Geometry: final body of the model. Coordinates: model frame, mm. Give positions to 0.01 mm unless a question says otherwise; leave off trailing zeros. Order: outer loops, then holes, each group sorted by start corner. A loop starts at its lowest first (then second) coordinate and runs counter-clockwise, first axis right, second up. Notation, with made-up numbers: (6, -38) -> (28, -38) arc R24 cw to (28, -15) -> close; hole circle Ø3 at (79, -26.75). An arc over 180 degrees is marked (long way). Write item = value, one per line.
```python
from build123d import *

# Parameters (mm, degrees)
SKETCH1_W                        = 250
SKETCH1_H                        = 250
BOSS_EXTRUDE1_DEPTH              = 50
SKETCH2_W                        = 40
SKETCH2_H                        = 100
SKETCH2_H_2                      = 50
CUT_EXTRUDE1_DEPTH               = 45
FILLET1_R                        = 5
FILLET2_R                        = 5
SKETCH5_R                        = 6.25
CUT_EXTRUDE2_DEPTH               = 22
FILLET5_R                        = 1.5
LPATTERN4_COUNT                  = 10
LPATTERN4_PITCH                  = 16.5
LPATTERN4_COUNT_DIR2             = 10
LPATTERN4_PITCH_DIR2             = 16.5
FILLET5_OF_LPATTERN4_R           = 1.5
CUT_EXTRUDE4_DEPTH               = 45
SKETCH8_W                        = 100
SKETCH8_H                        = 20
CUT_EXTRUDE5_DEPTH               = 30
FILLET6_R                        = 2.5
FILLET7_R                        = 2
SKETCH10_R                       = 13.5
CUT_EXTRUDE6_DEPTH               = 358.071421427
SKETCH4_W                        = 25
SKETCH4_H                        = 17.5
CUT_EXTRUDE7_DEPTH               = 10
VERRUNDUNG1_R                    = 2.5
SKIZZE2_W                        = 25
SKIZZE2_H                        = 5
AUFSATZ_LINEAR_AUSTRAGEN1_DEPTH  = 12.5
AUFSATZ_LINEAR_AUSTRAGEN2_DEPTH  = 10
SKIZZE11_W                       = 164
SKIZZE11_H                       = 164
SCHNITT_LINEAR_AUSTRAGEN6_DEPTH  = 10
SKIZZE12_W                       = 174
SKIZZE12_H                       = 174
SCHNITT_LINEAR_AUSTRAGEN7_DEPTH  = 2.5
SKIZZE13_R                       = 1.5
SCHNITT_LINEAR_AUSTRAGEN8_DEPTH  = 2.5
SKIZZE14_W                       = 10
SKIZZE14_H                       = 10
AUFSATZ_LINEAR_AUSTRAGEN3_DEPTH  = 45
SKIZZE16_W                       = 45
SKIZZE16_H                       = 250
SCHNITT_LINEAR_AUSTRAGEN9_DEPTH  = 358.071421427
SKIZZE17_R                       = 2.5
SCHNITT_LINEAR_AUSTRAGEN10_DEPTH = 5
SKIZZE18_W                       = 174.6
SKIZZE18_H                       = 174.6
SCHNITT_LINEAR_AUSTRAGEN11_DEPTH = 2.5
SKIZZE19_W                       = 165
SKIZZE19_H                       = 165
SCHNITT_LINEAR_AUSTRAGEN12_DEPTH = 2.5


with BuildPart() as part:
    # Sketch1 → Boss-Extrude1 (new body)
    with BuildSketch(Plane.XY):
        with Locations((-125, 125)):
            Rectangle(SKETCH1_W, SKETCH1_H)
    extrude(amount=BOSS_EXTRUDE1_DEPTH)

    # Sketch2 → Cut-Extrude1 (cut)
    with BuildSketch(Plane.XY.offset(50)):
        with Locations((-35, 170)):
            Rectangle(SKETCH2_W, SKETCH2_H)
        with Locations((-35, 70)):
            Rectangle(SKETCH2_W, SKETCH2_H_2)
    extrude(amount=-CUT_EXTRUDE1_DEPTH, mode=Mode.SUBTRACT)

    # Fillet1
    fillet1_edges = [part.edges().sort_by_distance(p)[0] for p in [
        (-55, 170, 50),
        (-35, 120, 50),
        (-15, 170, 50),
        (-35, 220, 50),
    ]]
    fillet(fillet1_edges, radius=FILLET1_R)

    # Fillet2
    fillet2_edges = [part.edges().sort_by_distance(p)[0] for p in [
        (-55, 70, 50),
        (-35, 45, 50),
        (-15, 70, 50),
        (-35, 95, 50),
    ]]
    fillet(fillet2_edges, radius=FILLET2_R)

    # Sketch5 → Cut-Extrude2 (cut)
    with BuildSketch(Plane.XY.offset(50)):
        with Locations((-225, 190)):
            Circle(SKETCH5_R)
    cut_extrude2 = extrude(amount=-CUT_EXTRUDE2_DEPTH, mode=Mode.SUBTRACT)

    # Fillet5
    fillet5_edges = [part.edges().sort_by_distance(p)[0] for p in [
        (-231.25, 190, 50),
    ]]
    fillet(fillet5_edges, radius=FILLET5_R)

    # LPattern4: Cut-Extrude2 10 × 10
    with Locations(*[(i * LPATTERN4_PITCH, -j * LPATTERN4_PITCH_DIR2, 0) for i in range(LPATTERN4_COUNT) for j in range(LPATTERN4_COUNT_DIR2) if (i, j) != (0, 0)]):
        add(cut_extrude2, mode=Mode.SUBTRACT)

    # Fillet5 of LPattern4
    fillet5_of_lpattern4_edges = [part.edges().sort_by_distance(p)[0] for p in [
        (-231.25, 173.5, 50),
        (-231.25, 157, 50),
        (-231.25, 140.5, 50),
        (-231.25, 124, 50),
        (-231.25, 107.5, 50),
        (-231.25, 91, 50),
        (-231.25, 74.5, 50),
        (-231.25, 58, 50),
        (-231.25, 41.5, 50),
        (-214.75, 190, 50),
        (-214.75, 173.5, 50),
        (-214.75, 157, 50),
        (-214.75, 140.5, 50),
        (-214.75, 124, 50),
        (-214.75, 107.5, 50),
        (-214.75, 91, 50),
        (-214.75, 74.5, 50),
        (-214.75, 58, 50),
        (-214.75, 41.5, 50),
        (-198.25, 190, 50),
        (-198.25, 173.5, 50),
        (-198.25, 157, 50),
        (-198.25, 140.5, 50),
        (-198.25, 124, 50),
        (-198.25, 107.5, 50),
        (-198.25, 91, 50),
        (-198.25, 74.5, 50),
        (-198.25, 58, 50),
        (-198.25, 41.5, 50),
        (-181.75, 190, 50),
        (-181.75, 173.5, 50),
        (-181.75, 157, 50),
        (-181.75, 140.5, 50),
        (-181.75, 124, 50),
        (-181.75, 107.5, 50),
        (-181.75, 91, 50),
        (-181.75, 74.5, 50),
        (-181.75, 58, 50),
        (-181.75, 41.5, 50),
        (-165.25, 190, 50),
        (-165.25, 173.5, 50),
        (-165.25, 157, 50),
        (-165.25, 140.5, 50),
        (-165.25, 124, 50),
        (-165.25, 107.5, 50),
        (-165.25, 91, 50),
        (-165.25, 74.5, 50),
        (-165.25, 58, 50),
        (-165.25, 41.5, 50),
        (-148.75, 190, 50),
        (-148.75, 173.5, 50),
        (-148.75, 157, 50),
        (-148.75, 140.5, 50),
        (-148.75, 124, 50),
        (-148.75, 107.5, 50),
        (-148.75, 91, 50),
        (-148.75, 74.5, 50),
        (-148.75, 58, 50),
        (-148.75, 41.5, 50),
        (-132.25, 190, 50),
        (-132.25, 173.5, 50),
        (-132.25, 157, 50),
        (-132.25, 140.5, 50),
        (-132.25, 124, 50),
        (-132.25, 107.5, 50),
        (-132.25, 91, 50),
        (-132.25, 74.5, 50),
        (-132.25, 58, 50),
        (-132.25, 41.5, 50),
        (-115.75, 190, 50),
        (-115.75, 173.5, 50),
        (-115.75, 157, 50),
        (-115.75, 140.5, 50),
        (-115.75, 124, 50),
        (-115.75, 107.5, 50),
        (-115.75, 91, 50),
        (-115.75, 74.5, 50),
        (-115.75, 58, 50),
        (-115.75, 41.5, 50),
        (-99.25, 190, 50),
        (-99.25, 173.5, 50),
        (-99.25, 157, 50),
        (-99.25, 140.5, 50),
        (-99.25, 124, 50),
        (-99.25, 107.5, 50),
        (-99.25, 91, 50),
        (-99.25, 74.5, 50),
        (-99.25, 58, 50),
        (-99.25, 41.5, 50),
        (-82.75, 190, 50),
        (-82.75, 173.5, 50),
        (-82.75, 157, 50),
        (-82.75, 140.5, 50),
        (-82.75, 124, 50),
        (-82.75, 107.5, 50),
        (-82.75, 91, 50),
        (-82.75, 74.5, 50),
        (-82.75, 58, 50),
        (-82.75, 41.5, 50),
    ]]
    fillet(fillet5_of_lpattern4_edges, radius=FILLET5_OF_LPATTERN4_R)

    # Sketch7 → Cut-Extrude4 (cut)
    with BuildSketch(Plane(origin=(0, 0, 0), x_dir=(-1, 0, 0), z_dir=(0, 0, -1))):
        Polygon((5, 245), (245, 245), (245, 5), (5, 5), (5, 40), (60, 40), (60, 100), (5, 100), (5, 115), (60, 115), (60, 225), (5, 225), align=None)
    extrude(amount=-CUT_EXTRUDE4_DEPTH, mode=Mode.SUBTRACT)

    # Sketch8 → Cut-Extrude5 (cut)
    with BuildSketch(Plane.XY.offset(50)):
        with Locations((-125, 240)):
            Rectangle(SKETCH8_W, SKETCH8_H)
    extrude(amount=-CUT_EXTRUDE5_DEPTH, mode=Mode.SUBTRACT)

    # Fillet6
    fillet6_edges = [part.edges().sort_by_distance(p)[0] for p in [
        (-125, 230, 45),
        (-125, 230, 50),
    ]]
    fillet(fillet6_edges, radius=FILLET6_R - 0.0001)  # a hair under: the kernel refuses the full size

    # Fillet7
    fillet7_edges = [part.edges().sort_by_distance(p)[0] for p in [
        (-125, 245, 20),
        (-125, 250, 20),
    ]]
    fillet(fillet7_edges, radius=FILLET7_R)

    # Sketch10 → Cut-Extrude6 (cut, through all)
    with BuildSketch(Plane.XY.offset(50)):
        with Locations((-35, 20)):
            Circle(SKETCH10_R)
    extrude(amount=-CUT_EXTRUDE6_DEPTH, mode=Mode.SUBTRACT)

    # Sketch4 → Cut-Extrude7 (cut)
    with BuildSketch(Plane.XY.offset(50)):
        with Locations((-187.5, 241.25)):
            Rectangle(SKETCH4_W, SKETCH4_H)
        with Locations((-62.5, 241.25)):
            Rectangle(SKETCH4_W, SKETCH4_H)
    extrude(amount=-CUT_EXTRUDE7_DEPTH, mode=Mode.SUBTRACT)

    # Verrundung1
    verrundung1_edges = [part.edges().sort_by_distance(p)[0] for p in [
        (-48.5, 20, 45),
        (-48.5, 20, 50),
    ]]
    fillet(verrundung1_edges, radius=VERRUNDUNG1_R - 0.0001)  # a hair under: the kernel refuses the full size

    # Skizze2 → Aufsatz-Linear austragen1 (add)
    with BuildSketch(Plane.XZ.offset(-245)):
        with Locations((-187.5, 37.5)):
            Rectangle(SKIZZE2_W, SKIZZE2_H)
        with Locations((-62.5, 37.5)):
            Rectangle(SKIZZE2_W, SKIZZE2_H)
    extrude(amount=AUFSATZ_LINEAR_AUSTRAGEN1_DEPTH)

    # Skizze4 → Aufsatz-Linear austragen2 (add)
    with BuildSketch(Plane(origin=(0, 0, 45), x_dir=(-1, 0, 0), z_dir=(0, 0, -1))):
        Polygon((50, 232.5), (75, 232.5), (75, 227.5), (49, 227.5), (49, 245), (50, 245), align=None)
        Polygon((200, 232.5), (175, 232.5), (175, 227.5), (201, 227.5), (201, 245), (200, 245), align=None)
    extrude(amount=AUFSATZ_LINEAR_AUSTRAGEN2_DEPTH)

    # Skizze11 → Schnitt-Linear austragen6 (cut)
    with BuildSketch(Plane.XY.offset(50)):
        with Locations((-150.75, 115.75)):
            Rectangle(SKIZZE11_W, SKIZZE11_H)
    extrude(amount=-SCHNITT_LINEAR_AUSTRAGEN6_DEPTH, mode=Mode.SUBTRACT)

    # Skizze12 → Schnitt-Linear austragen7 (cut)
    with BuildSketch(Plane.XY.offset(50)):
        with Locations((-150.75, 115.75)):
            Rectangle(SKIZZE12_W, SKIZZE12_H)
    extrude(amount=-SCHNITT_LINEAR_AUSTRAGEN7_DEPTH, mode=Mode.SUBTRACT)

    # Skizze13 → Schnitt-Linear austragen8 (cut)
    with BuildSketch(Plane.XY.offset(47.5)):
        with Locations((-235.25, 200.25)):
            Circle(SKIZZE13_R)
        with Locations((-150.75, 200.25)):
            Circle(SKIZZE13_R)
        with Locations((-66.25, 200.25)):
            Circle(SKIZZE13_R)
        with Locations((-235.25, 115.75)):
            Circle(SKIZZE13_R)
        with Locations((-66.25, 115.75)):
            Circle(SKIZZE13_R)
        with Locations(Location((-66.25, 31.25, 0), (0, 0, 180))):
            Circle(SKIZZE13_R)
        with Locations(Location((-150.75, 31.25, 0), (0, 0, 180))):
            Circle(SKIZZE13_R)
        with Locations(Location((-235.25, 31.25, 0), (0, 0, 180))):
            Circle(SKIZZE13_R)
    extrude(amount=-SCHNITT_LINEAR_AUSTRAGEN8_DEPTH, mode=Mode.SUBTRACT)

    # Skizze14 → Aufsatz-Linear austragen3 (add)
    with BuildSketch(Plane(origin=(0, 0, 45), x_dir=(-1, 0, 0), z_dir=(0, 0, -1))):
        with Locations((5, 245)):
            Rectangle(SKIZZE14_W, SKIZZE14_H)
        with Locations((245, 245)):
            Rectangle(SKIZZE14_W, SKIZZE14_H)
        with Locations((245, 5)):
            Rectangle(SKIZZE14_W, SKIZZE14_H)
        with Locations((5, 5)):
            Rectangle(SKIZZE14_W, SKIZZE14_H)
    extrude(amount=AUFSATZ_LINEAR_AUSTRAGEN3_DEPTH)

    # Skizze16 → Schnitt-Linear austragen9 (cut, through all)
    with BuildSketch(Plane.ZY.offset(250)):
        with Locations((22.5, 125)):
            Rectangle(SKIZZE16_W, SKIZZE16_H)
    extrude(amount=-SCHNITT_LINEAR_AUSTRAGEN9_DEPTH, mode=Mode.SUBTRACT)

    # Skizze17 → Schnitt-Linear austragen10 (cut)
    with BuildSketch(Plane.XY.offset(50)):
        with Locations((-245, 245)):
            Circle(SKIZZE17_R)
        with Locations((-5, 245)):
            Circle(SKIZZE17_R)
        with Locations((-5, 5)):
            Circle(SKIZZE17_R)
        with Locations((-245, 5)):
            Circle(SKIZZE17_R)
    extrude(amount=-SCHNITT_LINEAR_AUSTRAGEN10_DEPTH, mode=Mode.SUBTRACT)

    # Skizze18 → Schnitt-Linear austragen11 (cut)
    with BuildSketch(Plane.XY.offset(50)):
        with Locations((-150.75, 115.75)):
            Rectangle(SKIZZE18_W, SKIZZE18_H)
    extrude(amount=-SCHNITT_LINEAR_AUSTRAGEN11_DEPTH, mode=Mode.SUBTRACT)

    # Skizze19 → Schnitt-Linear austragen12 (cut)
    with BuildSketch(Plane.XY.offset(47.5)):
        with Locations((-150.75, 115.75)):
            Rectangle(SKIZZE19_W, SKIZZE19_H)
    extrude(amount=-SCHNITT_LINEAR_AUSTRAGEN12_DEPTH, mode=Mode.SUBTRACT)


solid = part.part
```
1) Section query B-B (y = 180). Output: boundary loops of the cut face in (x, z), plus the area to 3 significant figures.
Check sheet entries:
outline = (-250, 45) -> (-233.25, 45) -> (-233.25, 47.5) -> (-238.05, 47.5) -> (-238.05, 50) -> (-250, 50) -> close; (-68.25, 45) -> (-55, 45) arc R5 ccw to (-60, 50) -> (-63.45, 50) -> (-63.45, 47.5) -> (-68.25, 47.5) -> close; (-15, 45) -> (0, 45) -> (0, 50) -> (-10, 50) arc R5 ccw to start
area = 190 mm²
2) Section query C-C (z = 48.35). Count the separate pieces of the cut face and the enclosed holes in it, plus the area to 3 significant figures.
Check sheet entries:
separate_pieces = 1
enclosed_holes = 8
area = 21,900 mm²
3) First-contact query: P1, Ø0.8, axis at x = -138.5, z = 48.5, coming from the -Y side; P2, Ø5, axis at x = -150.75, y = 200.25, coming from the +Z side; P3, Ø0.8, axis at x = -180, z = 48.5, coming from the +Y side; P4, Ø1.8, axis at x = -235.25, y = 115.75, coming from the -Z side. Flat tips, straight axial feed; report the tip coordinate or a pass-through.
Check sheet entries:
P1 = 0
P2 = 47.5
P3 = 232.5
P4 = through
4) Section query A-A (x = -209). Output: boundary loops of the cut face in (y, z).
Check sheet entries:
outline = (0, 45) -> (33.25, 45) -> (33.25, 47.5) -> (28.45, 47.5) -> (28.45, 50) -> (0, 50) -> close; (198.25, 45) -> (250, 45) -> (250, 50) -> (203.05, 50) -> (203.05, 47.5) -> (198.25, 47.5) -> close
5) Mould query, pull axis X, two halves, no side actions, for faces 1 (the face through (-61, 135, 50)), 2 (the face through (-158, 32, 47.5)). Classes: +X half, -X half, draft (parallel to the pull), parting line (faces both ways), or undercut.
Check sheet entries:
face_1 = draft
face_2 = undercut
6) Line query: line 1 (Y direction, x = -5, z = 48.9); line 2 (X direction, y = 48, z = 45.5); line 3 (Y direction, x = -66.25, z = 46.8). Output: solid intervals per line, ascending. Write a range as from..to.
Check sheet entries:
line_1 = 0..2.5, 7.5..242.5, 247.5..250
line_2 = -250..-233.25, -68.25..-55.03, -14.97..0
line_3 = 0..29.75, 32.75..114.25, 117.25..198.75, 201.75..232.5
